Read the model definition and answer for the solid it produces. Units are mm, in the model's axes. A direction names the side the tool comes from. Coordinates: 2 decimals unless noted, no trailing zeros. Order: outer loops, then holes, each group sorted by start corner. A loop starts at its lowest first (then second) coordinate and runs counter-clockwise, first axis right, second up. Notation, with made-up numbers: (-36, 36) -> (1, 36) arc R35 ccw to (1, 73) -> close; hole circle Ø4 at (51.25, 61). An arc over 180 degrees is marked (long way). Answer as a JSON object with one key per item and string values. Group by question number.
1) Given pin 1 (8.5 mm diameter, centred on y = -1.5, z = -13, fed in from +X); pin 2 (7 mm diameter, centred on x = 13.5, y = 2.5, fed in from -Z); pin 3 (3 mm diameter, centred on x = 29, y = -6, fed in from +Z), each flat-ended and moving along its own axis, determine where each tip first touches the part or whether it passes through.
2) Consider L1, parallel to Z at x = 4.25, y = 11; L2, parallel to Y at x = 4.75, z = 16; L3, parallel to Z at x = 16.5, y = -8.75. Determine where each line is inside the solid, lowest interval first.
3) Determine the mould class of faces 6 (the cylindrical face through (36.034, -9.597, 12.939)), 7 (the cylindrical face through (3.796, 10.406, -22.568)), 8 (the flat face through (0, 0, 0)) for opening direction X: released by +X, released by -X, zero draft, split by the parting line, or undercut.
4) A tool of negligible diameter and unlimited length cuts with its end or side. For faces 1 (the flat face through (5, -14.25, 8)), 2 (the flat face through (34.2, 8, 11.4)), 3 (the flat face through (28.08, -0.2, 13.28)), 4 (the cylindrical face through (3.8, 10.06, 14.77)), 5 (the flat face through (30.45, 10.63, 13.01)), from which of +Z, -Z, +X, -X, +Y, -Y can it reach the whole face along a straight path? Write none if from no direction.
5) Section A-A on z = -24 is taken. Determine the outline of the cut face in (x, y).
6) Section B-B on x = 4.5 is taken. Determine the outline of the cut face in (y, z).
7) Section C-C on y = 10.25 is taken. Count the separate pieces of the cut face and the enclosed holes in it, and give its area (3 significant figures).
Solid Edge part; units mm, degrees
sketch "Sketch1" plane through (0, 0, 0) normal (1, 0, 0) x (0, 1, 0)
  line L0 (-14.25, -27.25) -> (-14.25, 27.25)
  line L1 (-14.25, 27.25) -> (14.25, 27.25)
  line L2 (14.25, 27.25) -> (14.25, -27.25)
  line L3 (14.25, -27.25) -> (-14.25, -27.25)
extrude "Protrusion1" add sketch "Sketch1" along normal blind 7.7
sketch "Sketch2" plane through (7.7, 0, 0) normal (1, 0, 0) x (0, 1, 0)
  line L0 (14.25, 19.55) -> (-14.25, 19.55)
  line L1 (-14.25, 19.55) -> (-14.25, 27.25)
  line L2 (-14.25, 27.25) -> (14.25, 27.25)
  line L3 (14.25, 27.25) -> (14.25, 19.55)
extrude "Extrusionsausprägung_2" add sketch "Sketch2" along normal blind 14.11
hole "Bohrung_1" at (0, 11, -24) direction (1, 0, 0) diameter 3.1 end through all
pattern_linear "Pattern1" count 2 spacing 22 along (0, -1, 0) count 2 spacing 40 along (0, 0, 1) of "Bohrung_1"
draft "Formschräge_3" angle 45 neutral plane through (18.75, 0, 19.55) normal (0, 0, -1) pull direction (0, 0, -1) face at (21.81, 9.215, 26.0437)
sketch "Sketch3" plane through (29.505, 0, 27.245) normal (0.7071068, 0, -0.7071068) x (0, 1, 0)
  line L0 (-14.25, -10.8824) -> (14.25, -10.8824)
  line L1 (14.25, -10.8824) -> (14.25, -3.1824)
  line L2 (14.25, -3.1824) -> (-14.25, -3.1824)
  line L3 (-14.25, -3.1824) -> (-14.25, -10.8824)
extrude "Extrusionsausprägung_3" add sketch "Sketch3" along normal blind 18
sketch "Sketch4" plane through (32.5061, -14.25, 0) normal (0, -1, 0) x (1, 0, 0)
  line L0 (-5.2514, 24.9947) -> (-7.5067, 27.25)
extrude "Cutout1" cut sketch "Sketch4" against normal through all material side at (26.1624, -14.25, 26.1577)
hole "Bohrung_10" at (31.123, -9.25, 10.237) direction (0.7071068, 0, 0.7071068) diameter 3.2 end up to next
hole "Hole1" at (31.123, 9.25, 10.237) direction (0.7071068, 0, 0.7071068) diameter 3.2 end up to next
sketch "Sketch5" plane through (28.8811, 0, 12.4789) normal (-0.7071068, 0, -0.7071068) x (0.7071068, 0, -0.7071068)
  line L0 (4.7872, 12.05) -> (1.554, 12.05)
  line L1 (1.554, 12.05) -> (-0.0626, 9.25)
  line L2 (-0.0626, 9.25) -> (1.554, 6.45)
  line L3 (1.554, 6.45) -> (4.7872, 6.45)
  line L4 (4.7872, 6.45) -> (6.4038, 9.25)
  line L5 (6.4038, 9.25) -> (4.7872, 12.05)
extrude "Extrusionsausschnitt_2" cut sketch "Sketch5" against normal blind 3
sketch "Sketch6" plane through (28.8811, 0, 12.4789) normal (-0.7071068, 0, -0.7071068) x (0.7071068, 0, -0.7071068)
  line L0 (4.7872, -12.05) -> (6.4038, -9.25)
  line L1 (6.4038, -9.25) -> (4.7872, -6.45)
  line L2 (4.7872, -6.45) -> (1.554, -6.45)
  line L3 (1.554, -6.45) -> (-0.0626, -9.25)
  line L4 (-0.0626, -9.25) -> (1.554, -12.05)
  line L5 (1.554, -12.05) -> (4.7872, -12.05)
extrude "Extrusionsausschnitt_3" cut sketch "Sketch6" against normal blind 3
hole "Hole2" [suppressed]
hole "Hole3" [suppressed]
properties material "PVC"
Worked answers:
{
 "1": {"pin 1": "stops at x = 7.7", "pin 2": "stops at z = 19.55", "pin 3": "stops at z = 24.75"},
 "2": {"L1": "z = -27.25 to -25.55, -22.45 to 14.45, 17.55 to 27.25", "L2": "y = -14.25 to -12.55, -9.45 to 9.45, 12.55 to 14.25", "L3": "z = 19.55 to 27.25"},
 "3": {"face 6": "undercut", "face 7": "zero draft", "face 8": "released by -X"},
 "4": {"face 1": "+Z, -Z, +X, -X, -Y", "face 2": "none", "face 3": "-Z, +Y, -Y", "face 4": "-X", "face 5": "-Z"},
 "5": {"outline": "(0, -14.25) -> (7.7, -14.25) -> (7.7, -12.55) -> (0, -12.55) -> close; (0, -9.45) -> (7.7, -9.45) -> (7.7, 9.45) -> (0, 9.45) -> close; (0, 12.55) -> (7.7, 12.55) -> (7.7, 14.25) -> (0, 14.25) -> close"},
 "6": {"outline": "(-14.25, -27.25) -> (14.25, -27.25) -> (14.25, 27.25) -> (-14.25, 27.25) -> close; hole circle Ø3.1 at (-11, -24); hole circle Ø3.1 at (-11, 16); hole circle Ø3.1 at (11, -24); hole circle Ø3.1 at (11, 16)"},
 "7": {"separate pieces": "4", "enclosed holes": "0", "area": "622 mm²"}
}
